The listing builds one solid part. Answer for the finished solid, in the listing's coordinates (mm). Face numbers are marked on the shaded views. A direction names the side the tool comes from. Give positions to 0.01 mm unless a question says otherwise; leave off trailing zeros. Order: outer loops, then holes, each group sorted by start corner. A loop starts at its lowest first (then second) coordinate and runs counter-clockwise, first axis right, second up. Notation, with made-up numbers: (-35, 25.5) -> (-1, 25.5) arc R15 ccw to (-1, 42.5) -> close; hole circle Ø7 at (57.5, -13). An arc over 180 degrees is marked (long way). Write item = value, one per line. Start each with the question number.
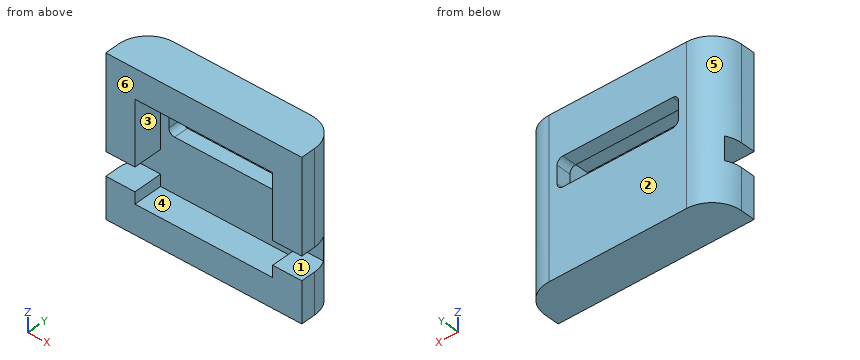
```python
from build123d import *

# Parameters (mm, degrees)
F1_DEPTH = 34.29
F2_W     = 29.972
F2_H     = 6.35
F3_DEPTH = 6.35
F2_W_2   = 6.35
F2_H_2   = 5.08
F2_W_3   = 36.322
F4_DEPTH = 6.35
F5_DEPTH = 9.526


with BuildPart() as f1:
    # F0 (on Top) → F1 (new body)
    with BuildSketch(Plane.XY):
        with BuildLine():
            Line((-21.336, -3.175), (-14.986, -3.175))
            Line((-14.986, -3.175), (-14.986, 3.175))
            Line((-14.986, 3.175), (14.986, 3.175))
            Line((14.986, 3.175), (14.986, -3.175))
            Line((14.986, -3.175), (21.336, -3.175))
            Line((21.336, -3.175), (21.336, 0))
            ThreePointArc((21.336, 0), (19.476128, 4.490128), (14.986, 6.35))
            Line((14.986, 6.35), (-14.986, 6.35))
            ThreePointArc((-14.986, 6.35), (-19.476128, 4.490128), (-21.336, 0))
            Line((-21.336, 0), (-21.336, -3.175))
        make_face()
    extrude(amount=F1_DEPTH)

    # F2 (on face) → F3 (join, through all)
    with BuildSketch(Plane.XZ.offset(3.175)):
        with Locations((0, 3.175)):
            Rectangle(F2_W, F2_H)
        with Locations((0, 31.115)):
            Rectangle(F2_W, F2_H)
    extrude(amount=-F3_DEPTH)

    # F2 (on face) → F4 (cut, through all)
    with BuildSketch(Plane.XZ.offset(3.175)):
        with Locations((-18.161, 11.43)):
            Rectangle(F2_W_2, F2_H_2)
        with Locations((3.175, 11.43)):
            Rectangle(F2_W_3, F2_H_2)
    extrude(amount=-F4_DEPTH, mode=Mode.SUBTRACT)

    # F2 (on face) → F5 (cut, through all)
    with BuildSketch(Plane.XZ.offset(3.175)):
        with BuildLine():
            ThreePointArc((-13.208, 19.304), (-12.836026, 18.405974), (-11.938, 18.034))
            Line((-11.938, 18.034), (0, 18.034))
            Line((0, 18.034), (11.938, 18.034))
            ThreePointArc((11.938, 18.034), (12.836026, 18.405974), (13.208, 19.304))
            Line((13.208, 19.304), (13.208, 23.114))
            ThreePointArc((13.208, 23.114), (12.836026, 24.012026), (11.938, 24.384))
            Line((11.938, 24.384), (-11.938, 24.384))
            ThreePointArc((-11.938, 24.384), (-12.836026, 24.012026), (-13.208, 23.114))
            Line((-13.208, 23.114), (-13.208, 19.304))
        make_face()
    extrude(amount=-F5_DEPTH, mode=Mode.SUBTRACT)


solid = f1.part
```
Item 1: Flat-ended cylindrical pins translate along their axes: pin 1 (1.5 mm diameter, centred on x = 11.5, z = 6.5, fed in from -Y) (3 decimals); pin 2 (2.5 mm diameter, centred on y = 5, z = 20.5, fed in from +X); pin 3 (2 mm diameter, centred on y = 3, z = 16.5, fed in from -X); pin 4 (6.5 mm diameter, centred on x = 2.5, z = 13, fed in from -Y) (3 decimals). Find the tip coordinate at first contact, or state that the pin passes through.
Item 2: A cutting plane is placed at A-A, the plane x = -2. Write down the section's boundary in (y, z) (3 decimals).
Item 3: A cutting plane is placed at C-C, the plane y = 0.5. Write down the section's boundary in (x, z).
Item 4: Which of the six approach directions +Z, -Z, +X, -X, +Y, -Y give full straight-line access (tool end or side, diameter ignored) to the marked faces 1, 2 and 3?
Item 5: Consider L1, parallel to Z at x = -9, y = 5.5; L2, parallel to Z at x = 8, y = 0.75; L3, parallel to X at y = -1.25, z = 25.5. Determine where each line is inside the solid, lowest interval first. Write a range as from..to.
Item 6: The mould has two halves that part along X. Classify the marked faces 4, 5 and 6: +X half, -X half, draft (parallel to the pull), parting line (faces both ways), or undercut.
Item 7: A cutting plane is placed at B-B, the plane z = 21. Write down the section's boundary in (x, y) (3 decimals), plus the area to 3 significant figures.
Item 8: A cutting plane is placed at D-D, the plane z = 4. Write down the section's boundary in (x, y) (3 decimals).
Check values:
q1.pin_1 = -3.175
q1.pin_2 = 20.11
q1.pin_3 = -21.01
q1.pin_4 = 3.175
q2.outline = (-3.175, 0) -> (6.35, 0) -> (6.35, 18.034) -> (3.175, 18.034) -> (3.175, 6.35) -> (-3.175, 6.35) -> close; (-3.175, 27.94) -> (3.175, 27.94) -> (3.175, 24.384) -> (6.35, 24.384) -> (6.35, 34.29) -> (-3.175, 34.29) -> close
q3.outline = (-21.32, 0) -> (21.32, 0) -> (21.32, 8.89) -> (14.99, 8.89) -> (14.99, 6.35) -> (-14.99, 6.35) -> (-14.99, 8.89) -> (-21.32, 8.89) -> close; (-21.32, 13.97) -> (-14.99, 13.97) -> (-14.99, 27.94) -> (14.99, 27.94) -> (14.99, 13.97) -> (21.32, 13.97) -> (21.32, 34.29) -> (-21.32, 34.29) -> close
q4.face_1 = +X, -X, -Y
q4.face_2 = +Z, -Z, +X, -X, +Y
q4.face_3 = -Y
q5.L1 = 0..18.03, 24.38..34.29
q5.L2 = 0..6.35, 27.94..34.29
q5.L3 = -21.34..-14.99, 14.99..21.34
q6.face_4 = undercut
q6.face_5 = -X half
q6.face_6 = draft
q7.outline = (-21.336, -3.175) -> (-14.986, -3.175) -> (-14.986, 3.175) -> (-13.208, 3.175) -> (-13.208, 6.35) -> (-14.986, 6.35) arc R6.35 ccw to (-21.336, 0) -> close; (13.208, 3.175) -> (14.986, 3.175) -> (14.986, -3.175) -> (21.336, -3.175) -> (21.336, 0) arc R6.35 ccw to (14.986, 6.35) -> (13.208, 6.35) -> close
q7.area = 115 mm^2
q8.outline = (-21.336, -3.175) -> (21.336, -3.175) -> (21.336, 0) arc R6.35 ccw to (14.986, 6.35) -> (-14.986, 6.35) arc R6.35 ccw to (-21.336, 0) -> close
